```python
from build123d import *

# Parameters (mm, degrees)
F0_W     = 457.2
F0_H     = 304.8
F1_DEPTH = 228.6
F2_T     = -3.175
F4_D     = 8


with BuildPart() as f1:
    # F0 (on Top) → F1 (new body)
    with BuildSketch(Plane.XY):
        with Locations((228.6, -152.4)):
            Rectangle(F0_W, F0_H)
    extrude(amount=F1_DEPTH)

    # F2
    f2_openings = [f1.faces().sort_by_distance(p)[0] for p in [
        (228.6, -152.4, 228.6),
    ]]
    offset(amount=F2_T, openings=f2_openings)

    # F4 (through all)
    with Locations(Plane(origin=(0, 0, 0), x_dir=(0, -1, 0), z_dir=(-1, 0, 0))):
        with Locations((203.2, 177.8), (101.6, 177.8)):
            Hole(F4_D / 2)


solid = f1.part
```
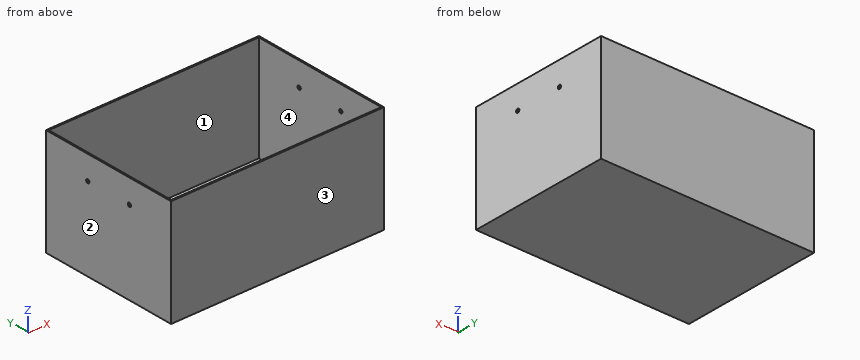
Part model, mm, in its own coordinate system. Face numbers are marked on the shaded views. Coordinates: 2 decimals unless noted, no trailing zeros. Write each loop counter-clockwise with the first axis right and the second up, starting at its lowest first coordinate (ties: lowest second). Pieces come first, ordered by that corner, then holes.
Item 1: Slice it at B-B (x = 423.5). Write the cut outline in (y, z) (3 decimals), and give its area (3 significant figures).
Item 2: Slice it at A-A (z = 213.5). Write the cut outline in (x, y) (3 decimals), and give its area (3 significant figures).
Item 3: Pin check, flat tips, straight feed: pin 1 (6.5 mm diameter, centred on y = -101.6, z = 177.8, fed in from +X); pin 2 (5 mm diameter, centred on x = 168, y = -47, fed in from +Z) (3 decimals). Stop position of each tip, or through.
Item 4: Probe line 1 (Y direction, x = 2, z = 177); line 2 (Z direction, x = 1, y = -203) (3 decimals); line 3 (Y direction, x = 198.5, z = 166.5) (3 decimals). List the from-to ranges inside material, lowest first.
Item 5: Slice it at C-C (y = -86). Write the cut outline in (x, z) (3 decimals).
Item 6: Mould opens along X. For the marked faces 1, 2, 3 and 4 say: released by +X, released by -X, zero draft, split by the parting line, or undercut.
Results found:
1. outline: (-304.8, 0) - (0, 0) - (0, 228.6) - (-3.175, 228.6) - (-3.175, 3.175) - (-301.625, 3.175) - (-301.625, 228.6) - (-304.8, 228.6) - close
1. area: 2,400 mm2
2. outline: (0, -304.8) - (457.2, -304.8) - (457.2, 0) - (0, 0) - close; hole (3.175, -301.625) - (454.025, -301.625) - (454.025, -3.175) - (3.175, -3.175) - close
2. area: 4,800 mm2
3. pin 1: passes through
3. pin 2: stops at z = 3.175
4. line 1: y = -304.8 to -207.12, -199.28 to -105.52, -97.68 to 0
4. line 2: z = 0 to 173.805, 181.795 to 228.6
4. line 3: y = -304.8 to -301.625, -3.175 to 0
5. outline: (0, 0) - (457.2, 0) - (457.2, 228.6) - (454.025, 228.6) - (454.025, 3.175) - (3.175, 3.175) - (3.175, 228.6) - (0, 228.6) - close
6. face 1: undercut
6. face 2: released by -X
6. face 3: zero draft
6. face 4: undercut
